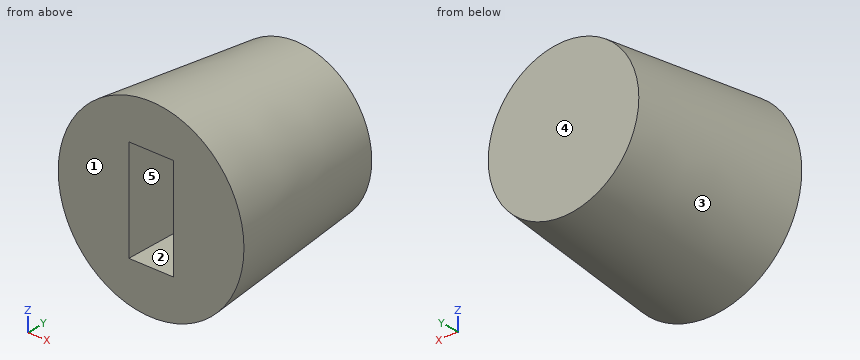
```python
from build123d import *

# Parameters (mm, degrees)
ESQUISSE2_R             = 5
BOSS_EXTRU_1_DEPTH      = 9
BOSS_EXTRU_1_TAPER      = 6
ESQUISSE3_W             = 2.4
ESQUISSE3_H             = 5.4
ENL_V_MAT_EXTRU_1_DEPTH = 7


with BuildPart() as part:
    # Esquisse2 → Boss.-Extru.1 (new body)
    with BuildSketch(Plane(origin=(0, 0, 0), x_dir=(1, 0, 0), z_dir=(0, 1, 0))):
        Circle(ESQUISSE2_R)
    extrude(amount=BOSS_EXTRU_1_DEPTH, taper=BOSS_EXTRU_1_TAPER)

    # Esquisse3 → Enlèv. mat.-Extru.1 (cut)
    with BuildSketch(Plane.XZ):
        Rectangle(ESQUISSE3_W, ESQUISSE3_H)
    extrude(amount=-ENL_V_MAT_EXTRU_1_DEPTH, mode=Mode.SUBTRACT)


solid = part.part
```
CAD build for the part. Positions are in the model's coordinates, mm. Face numbers are marked on the shaded views. A direction names the side the tool comes from. Coordinates: 2 decimals unless noted, no trailing zeros. Order: outer loops, then holes, each group sorted by start corner. A loop starts at its lowest first (then second) coordinate and runs counter-clockwise, first axis right, second up. Notation, with made-up numbers: (57.25, -10) -> (109.25, -10) arc R18 cw to (109.25, 6) -> close; hole circle Ø9 at (-38, -14.5). An arc over 180 degrees is marked (long way). Use one line per item in the form item = value. Start each with the question number.
1) Tool access for the marked faces 4 and 5: list every direction of +Z, -Z, +X, -X, +Y, -Y with a clear straight run to the whole face (end or side of a thin tool).
2) Pull direction Z, two halves, no side cores. Call the marked faces 1, 2 and 3: +Z half, -Z half, draft (parallel to the pull), parting line (faces both ways), or undercut.
3) Band-saw the part on A-A on x = 0. Give the cut face in (y, z).
4) Drop flat-ended pins along their axis: pin 1 (2.5 mm diameter, centred on x = 0, y = 2.5, fed in from +Z); pin 2 (2 mm diameter, centred on y = 2, z = 0.5, fed in from +X); pin 3 (1 mm diameter, centred on x = -3, y = 3.5, fed in from -Z). Give the stop position or say it passes through.
5) Drill centre lines: L1, parallel to Y at x = 1, z = 0; L2, parallel to X at y = 3, z = -0.5; L3, parallel to Z at x = -0.5, y = 3. Where is each one in solid material? Low to high. Write a range as [from, to].
6) Band-saw the part on B-B on y = 8.25. Give the cut face in (x, z), then the cut area to 3 significant figures.
Entries:
q1.face_4 = +Z, -Z, +X, -X, +Y
q1.face_5 = -Y
q2.face_1 = draft
q2.face_2 = undercut
q2.face_3 = parting line
q3.outline = (0, -5) -> (9, -4.05) -> (9, 4.05) -> (0, 5) -> (0, 2.7) -> (7, 2.7) -> (7, -2.7) -> (0, -2.7) -> close
q4.pin_1 = 4.87
q4.pin_2 = 4.89
q4.pin_3 = -3.91
q5.L1 = [7, 9]
q5.L2 = [-4.66, -1.2], [1.2, 4.66]
q5.L3 = [-4.66, -2.7], [2.7, 4.66]
q6.outline = circle Ø8.27 at (0, 0)
q6.area = 53.7 mm2
